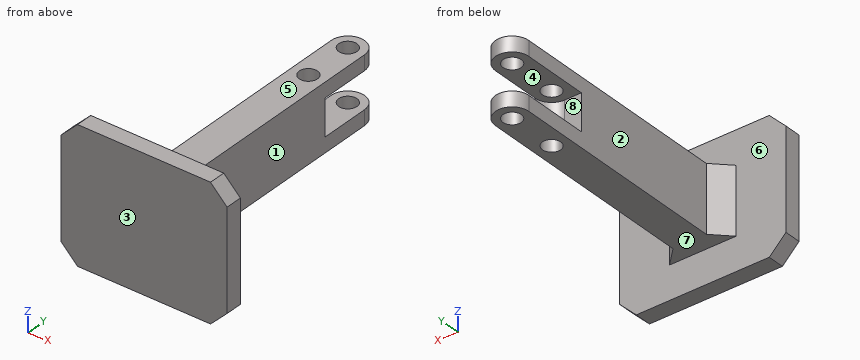
from build123d import *

# Parameters (mm, degrees)
BOSS_EXTRUDE1_DEPTH  = 10
M5_CLEARANCE_HOLE1_D = 5.5
CUT_EXTRUDE1_DEPTH   = 5.5
SKETCH1_4_W          = 50
SKETCH1_4_H          = 5
BOSS_EXTRUDE2_DEPTH  = 20
CHAMFER1_SIZE        = 5


with BuildPart() as part:
    # Sketch1 → Boss-Extrude1 (new body, symmetric)
    with BuildSketch(Plane.XY):
        with BuildLine():
            Line((-5, -65), (-25, -65))
            Line((-25, -65), (-25, -70))
            Line((-25, -70), (25, -70))
            Line((25, -70), (25, -65))
            Line((25, -65), (5, -65))
            Line((5, -65), (5, 7.5))
            ThreePointArc((5, 7.5), (0, 12.5), (-5, 7.5))
            Line((-5, 7.5), (-5, -65))
        make_face()
    extrude(amount=BOSS_EXTRUDE1_DEPTH, both=True)

    # M5 Clearance Hole1 (through all)
    with Locations(Plane.XY.offset(10)):
        with Locations((0, 7.5), (0, -7.5)):
            Hole(M5_CLEARANCE_HOLE1_D / 2)

    # Sketch1_3 → Cut-Extrude1 (cut, symmetric)
    with BuildSketch(Plane.XY):
        with BuildLine():
            ThreePointArc((0, -12.5), (3.535533906, -11.035533906), (5, -7.5))
            Line((5, -7.5), (5, 7.5))
            ThreePointArc((5, 7.5), (0, 12.5), (-5, 7.5))
            Line((-5, 7.5), (-5, -12.5))
            Line((-5, -12.5), (0, -12.5))
        make_face()
    extrude(amount=CUT_EXTRUDE1_DEPTH, both=True, mode=Mode.SUBTRACT)

    # Sketch1_4 → Boss-Extrude2 (add, symmetric)
    with BuildSketch(Plane.XY):
        with Locations((0, -67.5)):
            Rectangle(SKETCH1_4_W, SKETCH1_4_H)
    extrude(amount=BOSS_EXTRUDE2_DEPTH, both=True)

    # Chamfer1
    chamfer1_edges = [part.edges().sort_by_distance(p)[0] for p in [
        (5, -65, 0),
        (-5, -65, 0),
        (-25, -67.5, -20),
        (25, -67.5, 20),
        (-25, -67.5, 20),
        (25, -67.5, -20),
    ]]
    chamfer(chamfer1_edges, length=CHAMFER1_SIZE)


solid = part.part
Source: CAD feature listing. Evaluate the final solid. Frame: model axes, mm. Face numbers are marked on the shaded views. A direction names the side the tool comes from. Coordinates: 2 decimals unless noted, no trailing zeros. Order: outer loops, then holes, each group sorted by start corner. A loop starts at its lowest first (then second) coordinate and runs counter-clockwise, first axis right, second up.
Item 1: Cut plane C-C (y = -54.5). Return loops of the section in (x, z), plus the area to 3 significant figures.
Output values:
outline: (-5, -10) - (5, -10) - (5, 10) - (-5, 10) - close
area: 200 mm2
Item 2: Cut plane D-D (x = -1). Return loops of the section in (y, z).
Output values:
outline: (-70, -20) - (-65, -20) - (-65, -10) - (-10.06, -10) - (-10.06, -5.5) - (-12.5, -5.5) - (-12.5, 5.5) - (-10.06, 5.5) - (-10.06, 10) - (-65, 10) - (-65, 20) - (-70, 20) - close; (-4.94, -10) - (4.94, -10) - (4.94, -5.5) - (-4.94, -5.5) - close; (-4.94, 5.5) - (4.94, 5.5) - (4.94, 10) - (-4.94, 10) - close; (10.06, -10) - (12.4, -10) - (12.4, -5.5) - (10.06, -5.5) - close; (10.06, 5.5) - (12.4, 5.5) - (12.4, 10) - (10.06, 10) - close
Item 3: Cut plane A-A (z = 6.5). Return loops of the section in (x, y).
Output values:
outline: (-25, -70) - (25, -70) - (25, -65) - (10, -65) - (5, -60) - (5, 7.5) arc R5 ccw to (-5, 7.5) - (-5, -60) - (-10, -65) - (-25, -65) - close; hole circle Ø5.5 at (0, -7.5); hole circle Ø5.5 at (0, 7.5)
Item 4: Cut plane B-B (x = 8). Return loops of the section in (y, z), plus the area to 3 significant figures.
Output values:
outline: (-70, -20) - (-65, -20) - (-65, -10) - (-63, -10) - (-63, 10) - (-65, 10) - (-65, 20) - (-70, 20) - close
area: 240 mm2
Item 5: First-contact query: P1, Ø1, axis at x = -16.5, z = 10.5, coming from the +Y side; P2, Ø11, axis at x = -1, y = 0.5, coming from the +Z side; P3, Ø6, axis at y = -19, z = -2.5, coming from the -X side; P4, Ø4.5, axis at x = 0, y = -7.5, coming from the +Z side. Flat tips, straight axial feed; report the tip coordinate or a pass-through.
Output values:
P1: stops at y = -65
P2: stops at z = 10
P3: stops at x = -5
P4: passes through
Item 6: Set-up query: the marked faces 1, 2, 3 and 4. Return all of +Z, -Z, +X, -X, +Y, -Y with unobstructed straight access to the full face (end or side cutting, diameter ignored); none if empty.
Output values:
face 1: +Z, -Z, +X, +Y
face 2: +Z, -Z, -X, +Y
face 3: +Z, -Z, +X, -X, -Y
face 4: -X, +Y
Item 7: Pull-direction query (Z, two-part tool) for the marked faces 5, 6, 7 and 8; classes: pulls with the +Z half, pulls with the -Z half, needs draft (parallel to the pull), parting line crosses it, or undercut.
Output values:
face 5: pulls with the +Z half
face 6: needs draft
face 7: pulls with the -Z half
face 8: undercut
Item 8: Material intervals for line 1 (Y direction, x = 0, z = -8); line 2 (Y direction, x = -20, z = -12.5); line 3 (Z direction, x = -1, y = -54), sorted ascending.
Output values:
line 1: y = -70 to -10.25, -4.75 to 4.75, 10.25 to 12.5
line 2: y = -70 to -65
line 3: z = -10 to 10
